```python
from build123d import *

# Parameters (mm, degrees)
F0_W     = 76.2
F0_H     = 127
F1_DEPTH = 12.7
F2_W     = 88.9
F2_H     = 38.1
F3_DEPTH = 38.1


with BuildPart() as f1:
    # F0 (on Top) → F1 (new body)
    with BuildSketch(Plane.XY):
        Rectangle(F0_W, F0_H)
    extrude(amount=F1_DEPTH)

    # F2 (on Right) → F3 (join)
    with BuildSketch(Plane.YZ):
        with Locations((0, 31.75)):
            Rectangle(F2_W, F2_H)
    extrude(amount=F3_DEPTH)


solid = f1.part
```
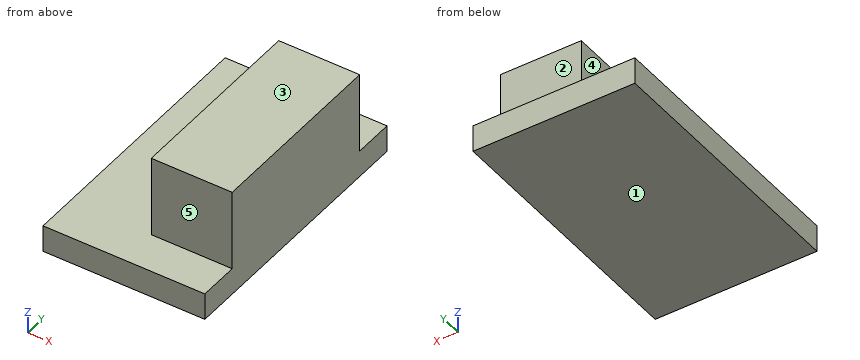
The model under review builds one solid part; all positions refer to its coordinate system, in mm. Face numbers are marked on the shaded views. A direction names the side the tool comes from. Give positions to 0.01 mm unless a question says otherwise; leave off trailing zeros. Write each loop counter-clockwise with the first axis right and the second up, starting at its lowest first coordinate (ties: lowest second). Pieces come first, ordered by that corner, then holes. Notation, with made-up numbers: (-39.5, 1.25) - (-10.5, 1.25) arc R14 cw to (-10.5, 9.25) - close; hole circle Ø6 at (55, 30). An arc over 180 degrees is marked (long way). Answer in a Markdown table with one row per item. Add a question column.
1. Tool access review of the marked faces 1, 2, 3, 4 and 5: name each direction out of +Z, -Z, +X, -X, +Y, -Y from which nothing blocks a thin tool from reaching the whole face with its end or side.
2. Wall thickness on line 1 along Y through (x, z) = (24, 32.5); line 2 along X through (y, z) = (25.5, 41); line 3 along Z through (x, y) = (-31.5, 53): over which ranges is each line inside the solid? List them lowest first. Write a range as [from, to].
3. We need section D-D on x = -22. Write out the cut boundary in (y, z), then the cut area to 3 significant figures.
4. We need section C-C on z = 45. Write out the cut boundary in (x, y).
5. Insertion check: P1, Ø5, axis at y = 8.5, z = 33.5, coming from the -X side; P2, Ø19, axis at x = 12, z = 23, coming from the +Y side; P3, Ø5, axis at x = 26.5, z = 18.5, coming from the -Y side. Each pin has a flat end and moves straight along its axis. Give the tip position at first contact, or say it passes through.
6. We need section A-A on x = 23. Write out the cut boundary in (y, z).
7. We need section B-B on y = 23.5. Write out the cut boundary in (x, z).
Ans:
| question | item | result |
|---|---|---|
| 1 | face 1 | -Z, +X, -X, +Y, -Y |
| 1 | face 2 | +Z, +X, -X, +Y |
| 1 | face 3 | +Z, +X, -X, +Y, -Y |
| 1 | face 4 | +Z, -X, +Y, -Y |
| 1 | face 5 | +Z, +X, -X, -Y |
| 2 | line 1 | y = [-44.45, 44.45] |
| 2 | line 2 | x = [0, 38.1] |
| 2 | line 3 | z = [0, 12.7] |
| 3 | outline | (-63.5, 0) - (63.5, 0) - (63.5, 12.7) - (-63.5, 12.7) - close |
| 3 | area | 1,610 mm^2 |
| 4 | outline | (0, -44.45) - (38.1, -44.45) - (38.1, 44.45) - (0, 44.45) - close |
| 5 | P1 | stops at x = 0 |
| 5 | P2 | stops at y = 44.45 |
| 5 | P3 | stops at y = -44.45 |
| 6 | outline | (-63.5, 0) - (63.5, 0) - (63.5, 12.7) - (44.45, 12.7) - (44.45, 50.8) - (-44.45, 50.8) - (-44.45, 12.7) - (-63.5, 12.7) - close |
| 7 | outline | (-38.1, 0) - (38.1, 0) - (38.1, 50.8) - (0, 50.8) - (0, 12.7) - (-38.1, 12.7) - close |
